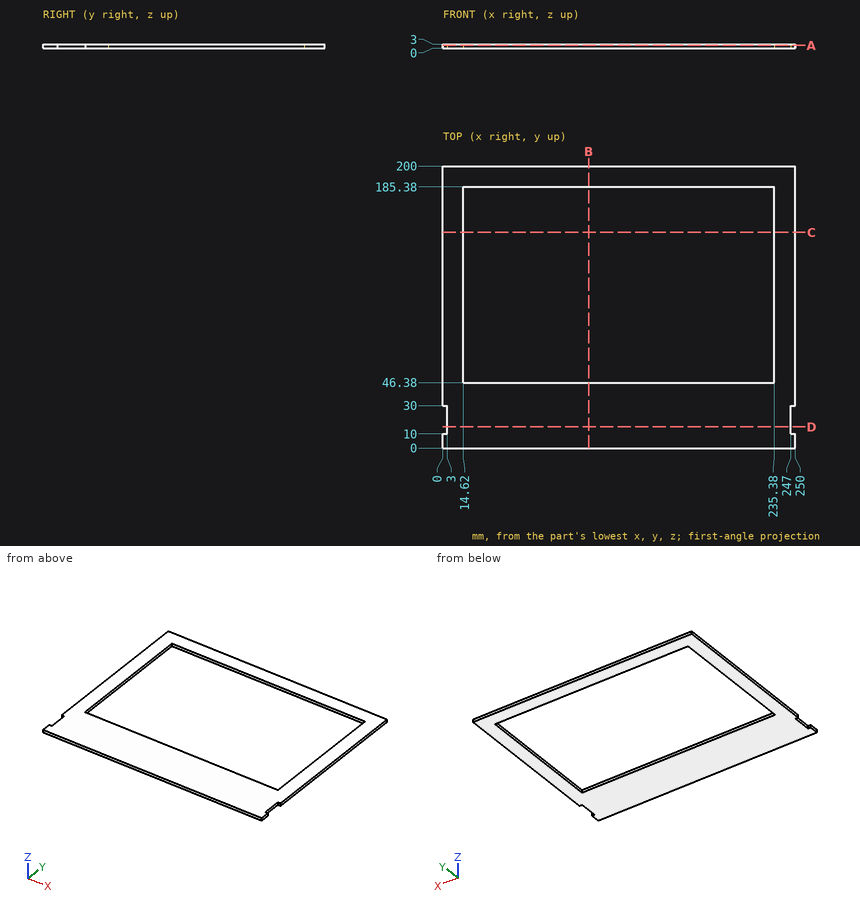
Print and shaded views of the part. All mm, measured from the part's lowest x, y and z. Give positions to 0.01 mm unless a question says otherwise; leave off trailing zeros. Loops run counter-clockwise (first coordinate to the right, second up) from the corner with the lowest first, then second, coordinate; pieces in that order, holes last. Notation, with made-up numbers: (33.5, -24) -> (84.5, -24) arc R10 cw to (84.5, -6) -> close; hole circle Ø2 at (38, 29). An arc over 180 degrees is marked (long way). Use a Markdown table: item, result.
1. Wall check: L1, parallel to Y at x = 37, z = 1.15; L2, parallel to X at y = 122.5, z = 2; L3, parallel to X at y = 19, z = 1.6. Give the ranges that are in metal, low to high. Write a range as [from, to].
Check result:
| item | result |
|---|---|
| L1 | y = [0, 46.38], [185.38, 200] |
| L2 | x = [0, 14.62], [235.38, 250] |
| L3 | x = [3, 247] |
2. Slice it at B-B (x = 103.5). List the corners of the cut face in (y, z).
Check result:
| item | result |
|---|---|
| outline | (0, 0) -> (46.38, 0) -> (46.38, 3) -> (0, 3) -> close; (185.38, 0) -> (200, 0) -> (200, 3) -> (185.38, 3) -> close |
3. Slice it at A-A (z = 2.05). List the corners of the cut face in (x, y), plus the area to 3 significant figures.
Check result:
| item | result |
|---|---|
| outline | (0, 0) -> (250, 0) -> (250, 10) -> (247, 10) -> (247, 30) -> (250, 30) -> (250, 200) -> (0, 200) -> (0, 30) -> (3, 30) -> (3, 10) -> (0, 10) -> close; hole (14.62, 46.38) -> (235.38, 46.38) -> (235.38, 185.38) -> (14.62, 185.38) -> close |
| area | 19,200 mm^2 |
4. Flat gauge pins, fed straight in: pin 1 (10 mm diameter, centred on x = 66.5, y = 176.5, fed in from -Z); pin 2 (1 mm diameter, centred on y = 22, z = 1, fed in from +X). Where does each tip first touch, or does it go through?
Check result:
| item | result |
|---|---|
| pin 1 | passes through |
| pin 2 | stops at x = 247 |
5. Slice it at D-D (y = 15). List the corners of the cut face in (x, z), plus the area to 3 significant figures.
Check result:
| item | result |
|---|---|
| outline | (3, 0) -> (247, 0) -> (247, 3) -> (3, 3) -> close |
| area | 732 mm^2 |
6. Slice it at C-C (y = 153). List the corners of the cut face in (x, z).
Check result:
| item | result |
|---|---|
| outline | (0, 0) -> (14.62, 0) -> (14.62, 3) -> (0, 3) -> close; (235.38, 0) -> (250, 0) -> (250, 3) -> (235.38, 3) -> close |
